The drawing under review shows one solid part. Ordinate dimensions are in mm from its lowest x, y, z. A direction names the side the tool comes from. Coordinates: 2 decimals unless noted, no trailing zeros. Order: outer loops, then holes, each group sorted by start corner. A loop starts at its lowest first (then second) coordinate and runs counter-clockwise, first axis right, second up.
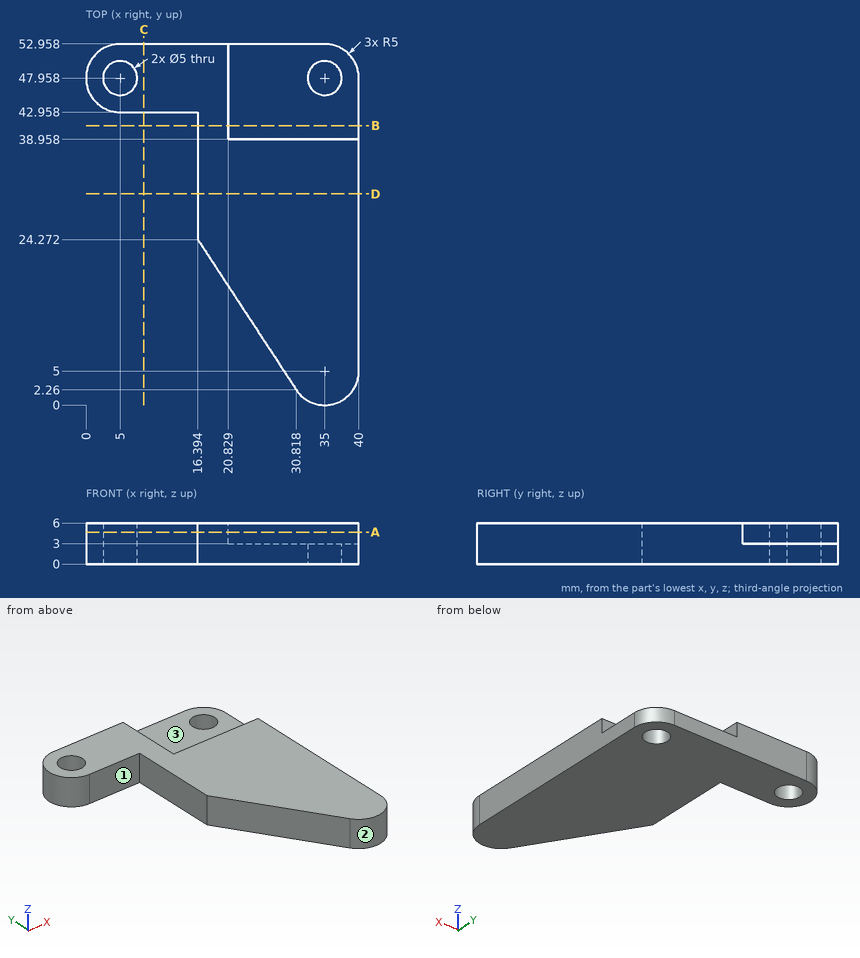
1. Machinability: for the marked faces 1, 2 and 3, which of the approach directions +Z, -Z, +X, -X, +Y, -Y give a long, thin tool a straight path to every point of the face, cutting with its end or side? Answer none if there is none.
Answer below:
face 1: +Z, -Z, -X, -Y
face 2: +Z, -Z, -Y
face 3: +Z, +X, +Y
2. Take a section at C-C, the plane x = 8.5. Give the boundary of the cut face in (y, z), plus the area to 3 significant figures.
Answer below:
outline: (42.96, 0) - (52.96, 0) - (52.96, 6) - (42.96, 6) - close
area: 60.0 mm2
3. Take a section at B-B, the plane y = 41. Give the boundary of the cut face in (x, z) (1 decimal).
Answer below:
outline: (16.4, 0) - (40, 0) - (40, 3) - (20.8, 3) - (20.8, 6) - (16.4, 6) - close
4. Take a section at D-D, the plane y = 31. Give the boundary of the cut face in (x, z) (1 decimal), plus the area to 3 significant figures.
Answer below:
outline: (16.4, 0) - (40, 0) - (40, 6) - (16.4, 6) - close
area: 142 mm2
5. To check wall thickness, follow L1, parallel to X at y = 48.5, z = 1.65; L2, parallel to Y at x = 5, z = 3.05; L3, parallel to Y at x = 35, z = 0.8. State the ranges of each line that lie inside material, in increasing order.
Answer below:
L1: x = 0.03 to 2.56, 7.44 to 32.56, 37.44 to 39.97
L2: y = 42.96 to 45.46, 50.46 to 52.96
L3: y = 0 to 45.46, 50.46 to 52.96
6. Take a section at A-A, the plane z = 4.7. Give the boundary of the cut face in (x, y) (1 decimal).
Answer below:
outline: (5, 43) - (16.4, 43) - (16.4, 24.3) - (30.8, 2.3) arc R5 ccw to (40, 5) - (40, 39) - (20.8, 39) - (20.8, 53) - (5, 53) arc R5 ccw to start; hole circle Ø5 at (5, 48)
7. Clearance check with flat-ended pins moving along their axes: pin 1 Ø1.5 at (y, z) = (49.5, 4.5) entering from +X; pin 2 Ø2 at (x, z) = (29.5, 0.5) entering from -Y (1 decimal); pin 3 Ø6 at (x, y) = (35, 47.96) entering from +Z; pin 4 Ø5 at (x, y) = (14.5, 46.5) entering from -Z. State where each tip first meets the part, or that it passes through.
Answer below:
pin 1: stops at x = 20.83
pin 2: stops at y = 2.7
pin 3: stops at z = 3
pin 4: stops at z = 0
